Here's how the part is built. I have some questions about the finished solid (model axes, mm). A direction names the side the tool comes from. Coordinates: 2 decimals unless noted, no trailing zeros. Write each loop counter-clockwise with the first axis right and the second up, starting at its lowest first coordinate (ties: lowest second). Pieces come first, ordered by that corner, then holes. Notation, with made-up numbers: M 8.25,54 L 15.25,54 A11 ccw 15.25,73 Z; hole C -24,64 d4. An arc over 180 degrees is marked long. Use a Markdown table: item, result.
Autodesk Inventor part; units mm, degrees
ref_plane "YZ Plane" through (0, 0, 0) normal (1, 0, 0) x (0, 1, 0)
ref_plane "XZ Plane" through (0, 0, 0) normal (0, 1, 0) x (-1, 0, 0)
ref_plane "XY Plane" through (0, 0, 0) normal (0, 0, 1) x (1, 0, 0)
sketch "Sketch1" plane through (0, 0, 0) normal (0, 0, 1) x (1, 0, 0)
  line L0 (0, 0) -> (75, 0)
  line L1 (75, 0) -> (75, -71.001)
  line L2 (75, -71.001) -> (0, -71.001)
  line L3 (0, -71.001) -> (0, 0)
  circle A0 centre (15, -29) radius 2.5
  circle A1 centre (25, -29) radius 2.5
  circle A2 centre (35, -29) radius 2.5
  circle A3 centre (25, -19) radius 2.5
  circle A4 centre (25, -39) radius 2.5
  circle A5 centre (4.85, -29) radius 2.5
  circle A6 centre (4.85, -39) radius 2.5
  circle A7 centre (4.85, -19) radius 2.5
  circle A8 centre (45.15, -19) radius 2.5
  circle A9 centre (45.15, -39) radius 2.5
  line L4 (0, 0) -> (50, 0)
  line L5 (50, 0) -> (50, -5)
  line L6 (0, -5) -> (0, 0)
  line L7 (0, -5) -> (75, -5)
  line L8 (0, -44) -> (75, -44)
  line L9 (0, -54) -> (75, -54)
  line L10 (0, -68) -> (75, -68)
  line L11 (0, -71) -> (75, -71)
  line L12 (45, -68) -> (45, -71)
  line L13 (6, -54) -> (6, -68)
  line L14 (0, -57) -> (6, -57)
  line L15 (0, -60) -> (6, -60)
  point P0 (37.5, 0)
  dimension "d0" = 75
  dimension "d1" = 71.001
  dimension "d3" = 5
  dimension "d4" = 10
  dimension "d6" = 10
  dimension "d8" = 10
  dimension "d10" = 10
  dimension "d12" = 20.15
  dimension "d15" = 20.15
  dimension "d23" = 5
  dimension "d29" = 39
  dimension "d30" = 15
  dimension "d31" = 10
  dimension "d44" = 14
  dimension "d45" = 3
  dimension "d46" = 25
  dimension "d52" = 30
  dimension "d69" = 6
  dimension "d71" = 3
  dimension "d72" = 3
sketch "Sketch1 outline for Extrusion1" plane through (0, 0, 0) normal (0, 0, 1) x (1, 0, 0)
  line L0 (75, 0) -> (0, 0)
  line L1 (0, 0) -> (0, -71.001)
  line L2 (0, -71.001) -> (75, -71.001)
  line L3 (75, -71.001) -> (75, 0)
  circle A0 centre (45.15, -19) radius 2.5
  circle A1 centre (4.85, -39) radius 2.5
  circle A2 centre (45.15, -39) radius 2.5
  circle A3 centre (4.85, -19) radius 2.5
extrude "Extrusion1" add sketch "Sketch1 outline for Extrusion1" along normal blind 6
sketch "Sketch1 outline for Extrusion3" plane through (0, 0, 0) normal (0, 0, 1) x (1, 0, 0)
  line L0 (75, 0) -> (0, 0)
  line L1 (75, -5) -> (75, 0)
  line L2 (0, -5) -> (75, -5)
  line L3 (0, 0) -> (0, -5)
  line L4 (75, -44) -> (0, -44)
  line L5 (75, -54) -> (75, -44)
  line L6 (0, -54) -> (75, -54)
  line L7 (0, -44) -> (0, -54)
extrude "Extrusion3" add sketch "Sketch1 outline for Extrusion3" along normal blind 54
sketch "Sketch3" plane through (0, 0, 0) normal (0, 1, 0) x (1, 0, 0)
  line L0 (0, -54) -> (75, -54)
  line L1 (0, 0) -> (75, 0)
  line L2 (75, 0) -> (75, -54)
  line L3 (75, -54) -> (0, -54)
  line L4 (0, -54) -> (0, 0)
  circle A0 centre (5.5, -48.5) radius 1.65
  circle A1 centre (36.5, -48.5) radius 1.65
  circle A2 centre (5.5, -17.5) radius 1.65
  circle A3 centre (36.5, -17.5) radius 1.65
  line L5 (21, -33) -> (21, -54) construction
  line L6 (18.4, -33) -> (18.4, -54)
  line L7 (23.6, -54) -> (23.6, -33)
  arc A4 (23.6, -33) -> (18.4, -33) centre (21, -33) ccw
  arc A5 (18.4, -54) -> (23.6, -54) centre (21, -54) ccw
  circle A6 centre (55, -44) radius 5
  point P0 (21, -43.5)
  dimension "d34" = 3.3
  dimension "d35" = 31
  dimension "d36" = 31
  dimension "d37" = 5.2
  dimension "d38" = 15.5
  dimension "d39" = 15.5
  dimension "d40" = 21
  dimension "d41" = 21
  dimension "d47" = 10
  dimension "d48" = 10
  dimension "d49" = 20
sketch "Sketch3 outline for Extrusion5" plane through (0, 0, 0) normal (0, 1, 0) x (1, 0, 0)
  arc A0 (23.6, -33) -> (18.4, -33) centre (21, -33) ccw
  line L0 (23.6, -54) -> (23.6, -33)
  arc A1 (18.4, -54) -> (23.6, -54) centre (21, -54) ccw
  line L1 (18.4, -33) -> (18.4, -54)
  circle A2 centre (5.5, -48.5) radius 1.65
  circle A3 centre (36.5, -48.5) radius 1.65
  circle A4 centre (5.5, -17.5) radius 1.65
  circle A5 centre (36.5, -17.5) radius 1.65
extrude "Extrusion5" cut sketch "Sketch3 outline for Extrusion5" against normal blind 5
sketch "Sketch3 outline for Extrusion6" plane through (0, 0, 0) normal (0, 1, 0) x (1, 0, 0)
  circle A0 centre (55, -44) radius 5
extrude "Extrusion6" cut sketch "Sketch3 outline for Extrusion6" against normal blind 54
sketch "Sketch1 outline for Extrusion7" plane through (0, 0, 0) normal (0, 0, 1) x (1, 0, 0)
  line L0 (75, -71) -> (75, -68)
  line L1 (45, -71) -> (75, -71)
  line L2 (45, -68) -> (45, -71)
  line L3 (75, -68) -> (45, -68)
extrude "Extrusion7" add sketch "Sketch1 outline for Extrusion7" along normal blind 32
sketch "Sketch4" plane through (45, -71, 6) normal (0, -1, 0) x (1, 0, 0)
  line L0 (0, 0) -> (30, 0)
  line L1 (0, 26) -> (30, 26)
  line L2 (0, 0) -> (30, 0)
  line L3 (30, 0) -> (30, 26)
  line L4 (30, 26) -> (0, 26)
  line L5 (0, 26) -> (0, 0)
  circle A0 centre (22.5, 24) radius 1
  circle A1 centre (22.5, 3) radius 1
  circle A2 centre (10, 3) radius 1
  circle A3 centre (10, 24) radius 1
  line L6 (0, 0) -> (0, 26)
  line L7 (15.5, 8) -> (4.5, 8)
  line L8 (4.5, 8) -> (4.5, 19)
  line L9 (4.5, 19) -> (15.5, 19)
  line L10 (15.5, 19) -> (15.5, 8)
  line L11 (15.5, 8) -> (4.5, 19) construction
  line L12 (4.5, 8) -> (15.5, 19) construction
  point P0 (-45, -6)
  point P1 (10, 13.5)
  point P2 (10, 13.5)
  point P3 (10, 13.5)
  dimension "d55" = 2
  dimension "d58" = 12.5
  dimension "d59" = 21
  dimension "d60" = 2
  dimension "d61" = 11
  dimension "d62" = 11
  dimension "d63" = 10.5
  dimension "d68" = 20
sketch "Sketch4 outline for Extrusion8" plane through (45, -71, 6) normal (0, -1, 0) x (1, 0, 0)
  line L0 (15.5, 8) -> (4.5, 8)
  line L1 (4.5, 8) -> (4.5, 19)
  line L2 (4.5, 19) -> (15.5, 19)
  line L3 (15.5, 19) -> (15.5, 8)
extrude "Extrusion8" cut sketch "Sketch4 outline for Extrusion8" against normal blind 3
sketch "Sketch4 outline for Extrusion9" plane through (45, -71, 6) normal (0, -1, 0) x (1, 0, 0)
  circle A0 centre (22.5, 24) radius 1
  circle A1 centre (22.5, 3) radius 1
  circle A2 centre (10, 3) radius 1
  circle A3 centre (10, 24) radius 1
extrude "Extrusion9" add sketch "Sketch4 outline for Extrusion9" against normal blind 6
sketch "Sketch1 outline for Extrusion10" plane through (0, 0, 0) normal (0, 0, 1) x (1, 0, 0)
  line L0 (6, -57) -> (0, -57)
  line L1 (6, -60) -> (6, -57)
  line L2 (0, -60) -> (6, -60)
  line L3 (0, -57) -> (0, -60)
extrude "Extrusion10" add sketch "Sketch1 outline for Extrusion10" along normal blind 26
sketch "Sketch5" plane through (0, -60, 6) normal (0, -1, 0) x (1, 0, 0)
  line L0 (6, 20) -> (0, 20)
  line L1 (0, -1.548307) -> (6, -1.548307)
  line L2 (6, -1.548307) -> (6, 20)
  line L3 (6, 20) -> (0, 20)
  line L4 (0, 20) -> (0, -1.548307)
  line L5 (0, 17) -> (6, 17)
  point P0 (0, -6)
  dimension "d75" = 3
sketch "Sketch5 outline for Extrusion11" plane through (0, -60, 6) normal (0, -1, 0) x (1, 0, 0)
  line L0 (6, 17) -> (6, 20)
  line L1 (0, 17) -> (6, 17)
  line L2 (0, 20) -> (0, 17)
  line L3 (6, 20) -> (0, 20)
extrude "Extrusion11" add sketch "Sketch5 outline for Extrusion11" against normal blind 6
fillet "Fillet1" radius 0.75 7 edges at (6, -57, 14.5) (0, -57, 14.5) (0, -54, 14.5) (0, -55.5, 23) (0, -55.5, 6) (6, -55.5, 23) (45, -68, 19)
properties part number "pnp-head"
1. Which directions (+Z, -Z, +X, -X, +Y, -Y) give clear straight access to the entire face, cutting with the end or side of a thin tool? Please do faces 4 (the face through (60.5, -70, 20)), 5 (the face through (23.6, -2, 44)), 6 (the face through (35.284, -2.465, 47.385)), 7 (the face through (60, -69, 32)), 8 (the face through (37, -5, 30)).
Answers follow:
| item | result |
|---|---|
| face 4 | -Y |
| face 5 | +Z, +Y |
| face 6 | +Y |
| face 7 | +Z, +X, -X, -Y |
| face 8 | +Z, +X, -X |
2. Suppose I cut it at A-A on y = -55. Write out the boundary of the cut face in (x, z).
Answers follow:
| item | result |
|---|---|
| outline | M 0,0 L 75,0 L 75,6 L 0.75,6 A0.75 ccw 0,5.25 Z; M 0,23.75 A0.75 ccw 0.75,23 L 5.25,23 A0.75 ccw 6,23.75 L 6,26 L 0,26 Z |
3. Will these pins go through, and if not, where does the flat tip stop? pin 1 Ø5 at (x, z) = (1.5, 21) entering from -Y; pin 2 Ø3 at (x, y) = (43, -16.5) entering from +Z; pin 3 Ø3 at (x, z) = (42.5, 40) entering from -Y.
Answers follow:
| item | result |
|---|---|
| pin 1 | stops at y = -60 |
| pin 2 | stops at z = 6 |
| pin 3 | stops at y = -54 |
4. Suppose I cut it at C-C on z = 37.5. Write out the boundary of the cut face in (x, y), and give its area (3 significant figures).
Answers follow:
| item | result |
|---|---|
| outline | M 0,-54 L 75,-54 L 75,-44 L 0,-44 Z; M 0,-5 L 18.4,-5 L 18.4,0 L 0,0 Z; M 23.6,-5 L 75,-5 L 75,0 L 23.6,0 Z |
| area | 1,100 mm2 |
5. Suppose I cut it at B-B on x = 36.5. Write out the boundary of the cut face in (y, z), and give its area (3 significant figures).
Answers follow:
| item | result |
|---|---|
| outline | M -71,0 L 0,0 L 0,15.85 L -5,15.85 L -5,6 L -44,6 L -44,54 L -54,54 L -54,6 L -71,6 Z; M -5,19.15 L 0,19.15 L 0,46.85 L -5,46.85 Z; M -5,50.15 L 0,50.15 L 0,54 L -5,54 Z |
| area | 1,110 mm2 |
6. I need wall thicknesses on probe 1 along X at (y, z) = (-3.15, 17.5); probe 2 along Y at (x, z) = (62, 25); probe 3 along Y at (x, z) = (4.85, 3.5). Which ranges of each line are inside material? Lowest first, please.
Answers follow:
| item | result |
|---|---|
| probe 1 | x = 0 to 3.85, 7.15 to 34.85, 38.15 to 75 |
| probe 2 | y = -71 to -68, -54 to -44, -5 to 0 |
| probe 3 | y = -71 to -41.5, -36.5 to -21.5, -16.5 to 0 |
7. Suppose I cut it at D-D on z = 44. Write out the boundary of the cut face in (x, y), and give its area (3 significant figures).
Answers follow:
| item | result |
|---|---|
| outline | M 0,-54 L 50,-54 L 50,-44 L 0,-44 Z; M 0,-5 L 18.4,-5 L 18.4,0 L 0,0 Z; M 23.6,-5 L 50,-5 L 50,0 L 23.6,0 Z; M 60,-54 L 75,-54 L 75,-44 L 60,-44 Z; M 60,-5 L 75,-5 L 75,0 L 60,0 Z |
| area | 949 mm2 |
8. We'd pull the mould along Z, two halves only. Please class faces 1 (the face through (49, -2, 54)), 2 (the face through (54.349, -2.465, 39.043)), 3 (the face through (6, -58, 18)): +Z half, -Z half, draft (parallel to the pull), parting line (faces both ways), or undercut.
Answers follow:
| item | result |
|---|---|
| face 1 | +Z half |
| face 2 | undercut |
| face 3 | draft |
